Geometry check sheet. Reference: the model listing, model coordinates, mm. Face numbers are marked on the shaded views. A direction names the side the tool comes from. Give positions to 0.01 mm unless a question says otherwise; leave off trailing zeros. Order: outer loops, then holes, each group sorted by start corner. A loop starts at its lowest first (then second) coordinate and runs counter-clockwise, first axis right, second up.
```python
from build123d import *

# Parameters (mm, degrees)
SKETCH1_R           = 8
SKETCH1_R_2         = 1.1
BOSS_EXTRUDE1_DEPTH = 2
BOSS_EXTRUDE2_DEPTH = 10


with BuildPart() as part:
    # Sketch1 → Boss-Extrude1 (new body)
    with BuildSketch(Plane.XY):
        Circle(SKETCH1_R)
        with Locations((-3.5, 0)):
            Circle(SKETCH1_R_2, mode=Mode.SUBTRACT)
        with Locations((1.75, 3.031088913)):
            Circle(SKETCH1_R_2, mode=Mode.SUBTRACT)
        with Locations((1.75, -3.031088913)):
            Circle(SKETCH1_R_2, mode=Mode.SUBTRACT)
    extrude(amount=BOSS_EXTRUDE1_DEPTH)

    # Sketch2 → Boss-Extrude2 (add)
    with BuildSketch(Plane.XY.offset(2)):
        with BuildLine():
            Line((-4.8, 4.5), (-5.361902647, 4.5))
            ThreePointArc((-5.361902647, 4.5), (-7, 0), (-5.361902647, -4.5))
            Line((-5.361902647, -4.5), (-4.8, -4.5))
            Line((-4.8, -4.5), (-4.8, 4.5))
        make_face()
        with BuildLine():
            ThreePointArc((7, 0), (6.577739678, 2.394439545), (5.361902647, 4.5))
            Line((5.361902647, 4.5), (4.8, 4.5))
            Line((4.8, 4.5), (4.8, -4.5))
            Line((4.8, -4.5), (5.361902647, -4.5))
            ThreePointArc((5.361902647, -4.5), (6.577739678, -2.394439545), (7, 0))
        make_face()
    extrude(amount=BOSS_EXTRUDE2_DEPTH)


solid = part.part
```
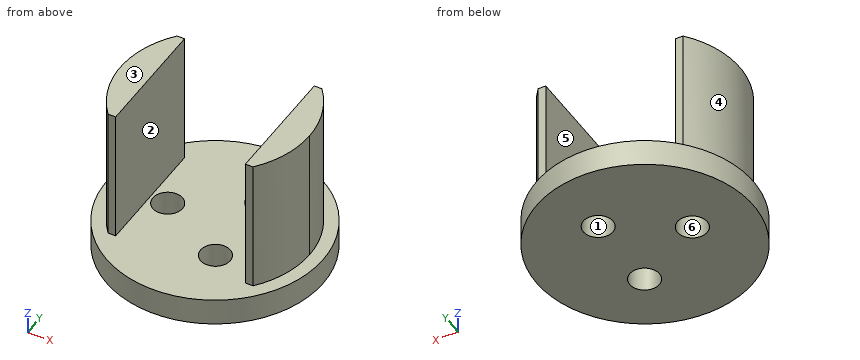
Q1. Cross-section at A-A, the plane z = 3.5. Record the boundary of the cut face in (x, y).
Q2. Gauge pin test, flat ends, axial feed: P1, Ø1.5, axis at y = 2.5, z = 9, coming from the -X side; P2, Ø1.5, axis at x = 3, y = -4, coming from the -Z side; P3, Ø5, axis at x = 5, z = 2.5, coming from the -Y side; P4, Ø2.5, axis at x = 1.75, y = -3.03, coming from the +Z side. Record the tip position at first contact, or that the pin passes through.
Q3. Thickness scan on L1, parallel to Y at x = 1.75, z = 0.8; L2, parallel to Z at x = -6.5, y = 3; L3, parallel to X at y = -2.5, z = 6. Record the ranges inside material, lowest first.
Q4. Cross-section at C-C, the plane x = -3.5. Record the boundary of the cut face in (y, z).
Q5. Cross-section at D-D, the plane y = -3.75. Record the boundary of the cut face in (x, z).
Q6. Access from +Z, -Z, +X, -X, +Y, -Y to the whole of each face (thin tool, end or side, straight path). Record for the marked faces 1 and 2.
Q7. Cross-section at B-B, the plane x = 1.5. Record the boundary of the cut face in (y, z).
Q8. Release check for a two-part mould opening along X. For the marked faces 3, 4, 5 and 6 record: pulls with the +X half, pulls with the -X half, needs draft (parallel to the pull), parting line crosses it, or undercut.
Answers follow:
1. outline: (-5.36, -4.5) - (-4.8, -4.5) - (-4.8, 4.5) - (-5.36, 4.5) arc R7 ccw to start; (4.8, -4.5) - (5.36, -4.5) arc R7 ccw to (5.36, 4.5) - (4.8, 4.5) - close
2. P1: stops at x = -6.78
2. P2: stops at z = 0
2. P3: stops at y = -7.58
2. P4: stops at z = 2
3. L1: y = -7.81 to -4.13, -1.93 to 1.93, 4.13 to 7.81
3. L2: z = 0 to 2
3. L3: x = -6.54 to -4.8, 4.8 to 6.54
4. outline: (-7.19, 0) - (-1.1, 0) - (-1.1, 2) - (-7.19, 2) - close; (1.1, 0) - (7.19, 0) - (7.19, 2) - (1.1, 2) - close
5. outline: (-7.07, 0) - (0.92, 0) - (0.92, 2) - (-4.8, 2) - (-4.8, 12) - (-5.91, 12) - (-5.91, 2) - (-7.07, 2) - close; (2.58, 0) - (7.07, 0) - (7.07, 2) - (5.91, 2) - (5.91, 12) - (4.8, 12) - (4.8, 2) - (2.58, 2) - close
6. face 1: +Z, -Z
6. face 2: +Z, +Y, -Y
7. outline: (-7.86, 0) - (-4.1, 0) - (-4.1, 2) - (-7.86, 2) - close; (-1.96, 0) - (1.96, 0) - (1.96, 2) - (-1.96, 2) - close; (4.1, 0) - (7.86, 0) - (7.86, 2) - (4.1, 2) - close
8. face 3: needs draft
8. face 4: pulls with the -X half
8. face 5: undercut
8. face 6: undercut
